Here's how the part is built. I have some questions about the finished solid (model axes, mm). Face numbers are marked on the shaded views. A direction names the side the tool comes from. Coordinates: 2 decimals unless noted, no trailing zeros. Write each loop counter-clockwise with the first axis right and the second up, starting at its lowest first coordinate (ties: lowest second). Pieces come first, ordered by that corner, then holes. Notation, with made-up numbers: M 65,-13 L 101,-13 A34 ccw 101,20 Z; hole C 13.5,21.25 d7. An arc over 180 degrees is marked long. Use one line per item in the form item = value. Start each with the question number.
1. I'm going to push flat-ended pins straight in: pin 1 Ø8.5 at (x, z) = (13, 7) entering from +Y; pin 2 Ø3.5 at (x, z) = (43, 6.5) entering from +Y; pin 3 Ø1 at (y, z) = (13.5, 8.5) entering from +X. Where does each tip first touch, or does it pass through?
2. I want a section at D-D, the plane y = 16.5. List the corners of the cut face in (x, z) for me.
3. I want a section at C-C, the plane x = 4.5. List the corners of the cut face in (y, z) for me, plus the area to 3 significant figures.
4. I want a section at B-B, the plane z = 5. List the corners of the cut face in (x, y) for me, plus the area to 3 significant figures.
5. On a 3-axis mill with a long thin cutter (end or side, diameter ignored), from which of +Z, -Z, +X, -X, +Y, -Y can I reach the whole of each face in a straight line? I mean the marked faces 1, 2 and 3. Say none if no direction works.
6. Please list where these lines run through material, in increasing order: line 1 along X through (y, z) = (31.4, 15); line 2 along Y through (x, z) = (3.5, 17.5). Write a range as [from, to].
7. I want a section at A-A, the plane x = -4. List the corners of the cut face in (y, z) for me.
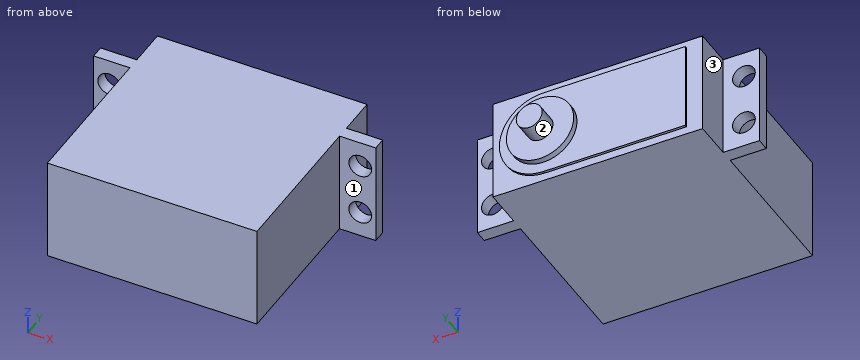
from build123d import *

# Parameters (mm, degrees)
SKETCH_1_W          = 40.5
SKETCH_1_H          = 20
EXTRUDE_1_DEPTH     = 30
SKETCH_2_W          = 54.5
SKETCH_2_H          = 20
EXTRUDE_2_DEPTH     = 2.5
SKETCH_3_W          = 40.5
SKETCH_3_H          = 20
EXTRUDE_3_DEPTH     = 7.5
EXTRUDE_4_DEPTH     = 0.5
SKETCH_5_R          = 6.5
EXTRUDE_5_DEPTH     = 1.2
SKETCH_6_R          = 2.5
EXTRUDE_6_DEPTH     = 3.95
SKETCH_7_R          = 2.2
CUT_EXTRUDE_1_DEPTH = 3.95


with BuildPart() as part:
    # 草图1 → 凸台-拉伸1 (new body)
    with BuildSketch(Plane(origin=(0, 0, 0), x_dir=(1, 0, 0), z_dir=(0, 1, 0))):
        with Locations((20.25, -10)):
            Rectangle(SKETCH_1_W, SKETCH_1_H)
    extrude(amount=EXTRUDE_1_DEPTH)

    # 草图2 → 凸台-拉伸2 (add)
    with BuildSketch(Plane(origin=(0, 30, 0), x_dir=(1, 0, 0), z_dir=(0, 1, 0))):
        with Locations((20.25, -10)):
            Rectangle(SKETCH_2_W, SKETCH_2_H)
    extrude(amount=EXTRUDE_2_DEPTH)

    # 草图3 → 凸台-拉伸3 (add)
    with BuildSketch(Plane(origin=(0, 32.5, 0), x_dir=(1, 0, 0), z_dir=(0, 1, 0))):
        with Locations((20.25, -10)):
            Rectangle(SKETCH_3_W, SKETCH_3_H)
    extrude(amount=EXTRUDE_3_DEPTH)

    # 草图4 → 凸台-拉伸4 (add)
    with BuildSketch(Plane(origin=(0, 40, 0), x_dir=(1, 0, 0), z_dir=(0, 1, 0))):
        with BuildLine():
            Line((3.073030725, -18.492151614), (30.5, -18.492151614))
            ThreePointArc((30.5, -18.492151614), (22.007848386, -10), (30.5, -1.507848386))
            Line((30.5, -1.507848386), (3.073030725, -1.507848386))
            Line((3.073030725, -1.507848386), (3.073030725, -18.492151614))
        make_face()
        with BuildLine():
            Line((30.5, -18.492151614), (30.5, -10))
            Line((30.5, -10), (30.5, -1.507848386))
            ThreePointArc((30.5, -1.507848386), (22.007848386, -10), (30.5, -18.492151614))
        make_face()
        with BuildLine():
            Line((30.5, -1.507848386), (30.5, -10))
            Line((30.5, -10), (38.992151614, -10))
            ThreePointArc((38.992151614, -10), (36.504857993, -3.995142007), (30.5, -1.507848386))
        make_face()
        with BuildLine():
            Line((38.992151614, -10), (30.5, -10))
            Line((30.5, -10), (30.5, -18.492151614))
            ThreePointArc((30.5, -18.492151614), (36.504857993, -16.004857993), (38.992151614, -10))
        make_face()
    extrude(amount=EXTRUDE_4_DEPTH)

    # 草图5 → 凸台-拉伸5 (add)
    with BuildSketch(Plane(origin=(0, 40.5, 0), x_dir=(1, 0, 0), z_dir=(0, 1, 0))):
        with Locations(Location((30.5, -10, 0), (0, 0, 270))):
            Circle(SKETCH_5_R)
    extrude(amount=EXTRUDE_5_DEPTH)

    # 草图6 → 凸台-拉伸6 (add)
    with BuildSketch(Plane(origin=(0, 41.7, 0), x_dir=(1, 0, 0), z_dir=(0, 1, 0))):
        with Locations(Location((30.5, -10, 0), (0, 0, 270))):
            Circle(SKETCH_6_R)
    extrude(amount=EXTRUDE_6_DEPTH)

    # 草图7 → 切除-拉伸1 (cut)
    with BuildSketch(Plane(origin=(0, 32.5, 0), x_dir=(1, 0, 0), z_dir=(0, 1, 0))):
        with Locations(Location((44.5, -5, 0), (0, 0, 270))):
            Circle(SKETCH_7_R)
        with Locations(Location((44.5, -15, 0), (0, 0, 270))):
            Circle(SKETCH_7_R)
        with Locations(Location((-4, -5, 0), (0, 0, 270))):
            Circle(SKETCH_7_R)
        with Locations(Location((-4, -15, 0), (0, 0, 270))):
            Circle(SKETCH_7_R)
    extrude(amount=-CUT_EXTRUDE_1_DEPTH, mode=Mode.SUBTRACT)


solid = part.part
Answer list:
q1.pin_1 = 40.5
q1.pin_2 = 32.5
q1.pin_3 = 40.5
q2.outline = M 0,0 L 40.5,0 L 40.5,20 L 0,20 Z
q3.outline = M 0,0 L 40,0 L 40,1.51 L 40.5,1.51 L 40.5,18.49 L 40,18.49 L 40,20 L 0,20 Z
q3.area = 808 mm²
q4.outline = M -7,30 L -6.2,30 L -6.2,32.5 L -7,32.5 Z; M -1.8,30 L 0,30 L 0,0 L 40.5,0 L 40.5,30 L 42.3,30 L 42.3,32.5 L 40.5,32.5 L 40.5,40 L 37.36,40 L 37.36,40.5 L 34.65,40.5 L 34.65,41.7 L 26.35,41.7 L 26.35,40.5 L 3.07,40.5 L 3.07,40 L 0,40 L 0,32.5 L -1.8,32.5 Z; M 46.7,30 L 47.5,30 L 47.5,32.5 L 46.7,32.5 Z
q4.area = 1,660 mm²
q5.face_1 = +Z, -Z, +X, -Y
q5.face_2 = +Y
q5.face_3 = +Z, -Z, -X, +Y
q6.line_1 = [-7, -6.2], [-1.8, 42.3], [46.7, 47.5]
q6.line_2 = [0, 40.5]
q7.outline = M 30,0 L 32.5,0 L 32.5,2.8 L 30,2.8 Z; M 30,7.2 L 32.5,7.2 L 32.5,12.8 L 30,12.8 Z; M 30,17.2 L 32.5,17.2 L 32.5,20 L 30,20 Z
